```python
from build123d import *

# Parameters (mm, degrees)
BOSS_EXTRUDE1_DEPTH = 5
SKETCH2_R           = 1.5
BOSS_EXTRUDE2_DEPTH = 6
CUT_EXTRUDE1_REACH  = 44.641
SKETCH3_R           = 1.5


with BuildPart() as part:
    # Sketch1 → Boss-Extrude1 (new body)
    with BuildSketch(Plane(origin=(0, 0, 0), x_dir=(1, 0, 0), z_dir=(0, 1, 0))):
        with BuildLine():
            Line((0, 0), (40, 0))
            Line((40, 0), (40, 12.3))
            Line((40, 12.3), (37.05, 12.3))
            ThreePointArc((37.05, 12.3), (36.84816772, 12.496593354), (36.725, 12.75))
            ThreePointArc((36.725, 12.75), (36.593980723, 13.132592289), (36.425, 13.5))
            Line((36.425, 13.5), (35.875, 13.5))
            ThreePointArc((35.875, 13.5), (35.706019277, 13.132592289), (35.575, 12.75))
            ThreePointArc((35.575, 12.75), (35.45183228, 12.496593354), (35.25, 12.3))
            Line((35.25, 12.3), (34.7, 12.3))
            ThreePointArc((34.7, 12.3), (34.49816772, 12.496593354), (34.375, 12.75))
            ThreePointArc((34.375, 12.75), (34.243980723, 13.132592289), (34.075, 13.5))
            Line((34.075, 13.5), (33.525, 13.5))
            ThreePointArc((33.525, 13.5), (33.356019277, 13.132592289), (33.225, 12.75))
            ThreePointArc((33.225, 12.75), (33.10183228, 12.496593354), (32.9, 12.3))
            Line((32.9, 12.3), (32.35, 12.3))
            ThreePointArc((32.35, 12.3), (32.14816772, 12.496593354), (32.025, 12.75))
            ThreePointArc((32.025, 12.75), (31.893980723, 13.132592289), (31.725, 13.5))
            Line((31.725, 13.5), (31.175, 13.5))
            ThreePointArc((31.175, 13.5), (31.006019277, 13.132592289), (30.875, 12.75))
            ThreePointArc((30.875, 12.75), (30.75183228, 12.496593354), (30.55, 12.3))
            Line((30.55, 12.3), (30, 12.3))
            ThreePointArc((30, 12.3), (29.79816772, 12.496593354), (29.675, 12.75))
            ThreePointArc((29.675, 12.75), (29.543980723, 13.132592289), (29.375, 13.5))
            Line((29.375, 13.5), (28.825, 13.5))
            ThreePointArc((28.825, 13.5), (28.656019277, 13.132592289), (28.525, 12.75))
            ThreePointArc((28.525, 12.75), (28.40183228, 12.496593354), (28.2, 12.3))
            Line((28.2, 12.3), (27.65, 12.3))
            ThreePointArc((27.65, 12.3), (27.44816772, 12.496593354), (27.325, 12.75))
            ThreePointArc((27.325, 12.75), (27.193980723, 13.132592289), (27.025, 13.5))
            Line((27.025, 13.5), (26.475, 13.5))
            ThreePointArc((26.475, 13.5), (26.306019277, 13.132592289), (26.175, 12.75))
            ThreePointArc((26.175, 12.75), (26.05183228, 12.496593354), (25.85, 12.3))
            Line((25.85, 12.3), (25.3, 12.3))
            ThreePointArc((25.3, 12.3), (25.09816772, 12.496593354), (24.975, 12.75))
            ThreePointArc((24.975, 12.75), (24.843980723, 13.132592289), (24.675, 13.5))
            Line((24.675, 13.5), (24.125, 13.5))
            ThreePointArc((24.125, 13.5), (23.956019277, 13.132592289), (23.825, 12.75))
            ThreePointArc((23.825, 12.75), (23.70183228, 12.496593354), (23.5, 12.3))
            Line((23.5, 12.3), (22.95, 12.3))
            ThreePointArc((22.95, 12.3), (22.74816772, 12.496593354), (22.625, 12.75))
            ThreePointArc((22.625, 12.75), (22.493980723, 13.132592289), (22.325, 13.5))
            Line((22.325, 13.5), (21.775, 13.5))
            ThreePointArc((21.775, 13.5), (21.606019277, 13.132592289), (21.475, 12.75))
            ThreePointArc((21.475, 12.75), (21.35183228, 12.496593354), (21.15, 12.3))
            Line((21.15, 12.3), (20.6, 12.3))
            ThreePointArc((20.6, 12.3), (20.39816772, 12.496593354), (20.275, 12.75))
            ThreePointArc((20.275, 12.75), (20.143980723, 13.132592289), (19.975, 13.5))
            Line((19.975, 13.5), (19.425, 13.5))
            ThreePointArc((19.425, 13.5), (19.256019277, 13.132592289), (19.125, 12.75))
            ThreePointArc((19.125, 12.75), (19.00183228, 12.496593354), (18.8, 12.3))
            Line((18.8, 12.3), (18.25, 12.3))
            ThreePointArc((18.25, 12.3), (18.04816772, 12.496593354), (17.925, 12.75))
            ThreePointArc((17.925, 12.75), (17.793980723, 13.132592289), (17.625, 13.5))
            Line((17.625, 13.5), (17.075, 13.5))
            ThreePointArc((17.075, 13.5), (16.906019277, 13.132592289), (16.775, 12.75))
            ThreePointArc((16.775, 12.75), (16.65183228, 12.496593354), (16.45, 12.3))
            Line((16.45, 12.3), (15.9, 12.3))
            ThreePointArc((15.9, 12.3), (15.69816772, 12.496593354), (15.575, 12.75))
            ThreePointArc((15.575, 12.75), (15.443980723, 13.132592289), (15.275, 13.5))
            Line((15.275, 13.5), (14.725, 13.5))
            ThreePointArc((14.725, 13.5), (14.556019277, 13.132592289), (14.425, 12.75))
            ThreePointArc((14.425, 12.75), (14.30183228, 12.496593354), (14.1, 12.3))
            Line((14.1, 12.3), (13.55, 12.3))
            ThreePointArc((13.55, 12.3), (13.34816772, 12.496593354), (13.225, 12.75))
            ThreePointArc((13.225, 12.75), (13.093980723, 13.132592289), (12.925, 13.5))
            Line((12.925, 13.5), (12.375, 13.5))
            ThreePointArc((12.375, 13.5), (12.206019277, 13.132592289), (12.075, 12.75))
            ThreePointArc((12.075, 12.75), (11.95183228, 12.496593354), (11.75, 12.3))
            Line((11.75, 12.3), (11.2, 12.3))
            ThreePointArc((11.2, 12.3), (10.99816772, 12.496593354), (10.875, 12.75))
            ThreePointArc((10.875, 12.75), (10.743980723, 13.132592289), (10.575, 13.5))
            Line((10.575, 13.5), (10.025, 13.5))
            ThreePointArc((10.025, 13.5), (9.856019277, 13.132592289), (9.725, 12.75))
            ThreePointArc((9.725, 12.75), (9.60183228, 12.496593354), (9.4, 12.3))
            Line((9.4, 12.3), (8.85, 12.3))
            ThreePointArc((8.85, 12.3), (8.64816772, 12.496593354), (8.525, 12.75))
            ThreePointArc((8.525, 12.75), (8.393980723, 13.132592289), (8.225, 13.5))
            Line((8.225, 13.5), (7.675, 13.5))
            ThreePointArc((7.675, 13.5), (7.506019277, 13.132592289), (7.375, 12.75))
            ThreePointArc((7.375, 12.75), (7.25183228, 12.496593354), (7.05, 12.3))
            Line((7.05, 12.3), (6.5, 12.3))
            ThreePointArc((6.5, 12.3), (6.29816772, 12.496593354), (6.175, 12.75))
            ThreePointArc((6.175, 12.75), (6.043980723, 13.132592289), (5.875, 13.5))
            Line((5.875, 13.5), (5.325, 13.5))
            ThreePointArc((5.325, 13.5), (5.156019277, 13.132592289), (5.025, 12.75))
            ThreePointArc((5.025, 12.75), (4.90183228, 12.496593354), (4.7, 12.3))
            Line((4.7, 12.3), (4.15, 12.3))
            ThreePointArc((4.15, 12.3), (3.94816772, 12.496593354), (3.825, 12.75))
            ThreePointArc((3.825, 12.75), (3.693980723, 13.132592289), (3.525, 13.5))
            Line((3.525, 13.5), (2.975, 13.5))
            ThreePointArc((2.975, 13.5), (2.806019277, 13.132592289), (2.675, 12.75))
            ThreePointArc((2.675, 12.75), (2.55183228, 12.496593354), (2.35, 12.3))
            Line((2.35, 12.3), (1.8, 12.3))
            ThreePointArc((1.8, 12.3), (1.59816772, 12.496593354), (1.475, 12.75))
            ThreePointArc((1.475, 12.75), (1.343980723, 13.132592289), (1.175, 13.5))
            Line((1.175, 13.5), (0.625, 13.5))
            ThreePointArc((0.625, 13.5), (0.456019277, 13.132592289), (0.325, 12.75))
            ThreePointArc((0.325, 12.75), (0.20183228, 12.496593354), (0, 12.3))
            Line((0, 12.3), (0, 0))
        make_face()
    extrude(amount=BOSS_EXTRUDE1_DEPTH)

    # Sketch2 → Boss-Extrude2 (add)
    # profile 1 of 2: a face of its own
    with BuildSketch(Plane.XZ):
        with BuildLine():
            Line((7, -7.5), (3, -7.5))
            ThreePointArc((3, -7.5), (0.5, -5), (3, -2.5))
            Line((3, -2.5), (7, -2.5))
            ThreePointArc((7, -2.5), (9.5, -5), (7, -7.5))
        make_face()
        with Locations(Location((5, -5, 0), (0, 0, 270))):
            Circle(SKETCH2_R, mode=Mode.SUBTRACT)
    # profile 2 of 2: a face of its own
    with BuildSketch(Plane.XZ):
        with BuildLine():
            Line((37, -7.5), (33, -7.5))
            ThreePointArc((33, -7.5), (30.5, -5), (33, -2.5))
            Line((33, -2.5), (37, -2.5))
            ThreePointArc((37, -2.5), (39.5, -5), (37, -7.5))
        make_face()
        with Locations(Location((35, -5, 0), (0, 0, 270))):
            Circle(SKETCH2_R, mode=Mode.SUBTRACT)
    extrude(amount=BOSS_EXTRUDE2_DEPTH)

    # Sketch3 → Cut-Extrude1 (cut, up to next)
    with BuildSketch(Plane.XZ, mode=Mode.PRIVATE) as cut_extrude1_sk1:
        with Locations(Location((35, -5, 0), (0, 0, 270))):
            Circle(SKETCH3_R)
    cut_extrude1_tool1 = extrude(cut_extrude1_sk1.sketch, amount=-CUT_EXTRUDE1_REACH, mode=Mode.PRIVATE) & part.part
    # Sketch3 → Cut-Extrude1 (cut, up to next)
    with BuildSketch(Plane.XZ, mode=Mode.PRIVATE) as cut_extrude1_sk2:
        with Locations(Location((5, -5, 0), (0, 0, 270))):
            Circle(SKETCH3_R)
    cut_extrude1_tool2 = extrude(cut_extrude1_sk2.sketch, amount=-CUT_EXTRUDE1_REACH, mode=Mode.PRIVATE) & part.part
    add(cut_extrude1_tool1.solids().sort_by_distance((35, 0, -5))[0], mode=Mode.SUBTRACT)
    add(cut_extrude1_tool2.solids().sort_by_distance((5, 0, -5))[0], mode=Mode.SUBTRACT)


solid = part.part
```
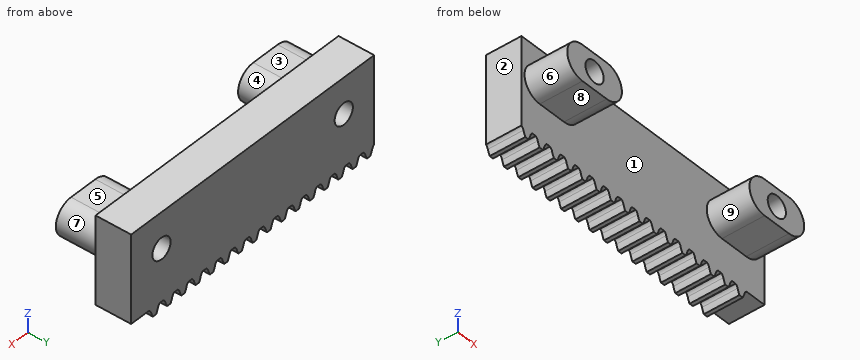
Check sheet for the modelled part. Datum: model origin and axes. Units: mm. Face numbers are marked on the shaded views. A direction names the side the tool comes from. Round coordinates to 2 decimals unless told otherwise and drop trailing zeros. Order: outer loops, then holes, each group sorted by start corner. A loop starts at its lowest first (then second) coordinate and runs counter-clockwise, first axis right, second up. Notation, with made-up numbers: (-27.5, 49) - (-6.5, 49) arc R25 cw to (-6.5, 82) - close; hole circle Ø8 at (39.5, 86). An arc over 180 degrees is marked (long way). Answer as CSV lines item,"result". Start each with the question number.
1) Scan lines: probe 1 along X at (y, z) = (2.55, -5); probe 2 along X at (y, z) = (-3.25, -5); probe 3 along X at (y, z) = (3.25, -6). Record each from-to range of solid material in increasing order.
2) Draft check along X on the marked faces 1, 2, 3 and 4. Enter one of: +X half, -X half, draft (parallel to the pull), parting line (faces both ways), or undercut.
3) Depth check by flat-ended pin: pin 1 (1.5 mm diameter, centred on x = 38, y = 2, fed in from -Z); pin 2 (2 mm diameter, centred on x = 35.5, y = -2.5, fed in from -Z); pin 3 (1.2 mm diameter, centred on x = 4.5, y = -2, fed in from +Z). Enter the tip coordinate at first touch or a pass-through.
4) Section check C-C (z = -10.25). Record the cut outline in (x, y), then the cut area to 3 significant figures.
5) Tool access check on the marked faces 5, 6, 7, 8 and 9. Record the directions out of +Z, -Z, +X, -X, +Y, -Y that give a thin tool (end or side, any length) a straight path to the whole face; none if there is none.
6) Section check A-A (y = -1.5). Record the cut outline in (x, z), then the cut area to 3 significant figures.
7) Section check D-D (x = 37.5). Record the cut outline in (y, z).
8) Section check B-B (z = -5). Record the cut outline in (x, y), then the cut area to 3 significant figures.
Determined:
1,probe 1,"0 to 3.5, 6.5 to 33.5, 36.5 to 40"
1,probe 2,"0.5 to 3.5, 6.5 to 9.5, 30.5 to 33.5, 36.5 to 39.5"
1,probe 3,"0 to 3.88, 6.12 to 33.88, 36.12 to 40"
2,face 1,"undercut"
2,face 2,"-X half"
2,face 3,"draft"
2,face 4,"undercut"
3,pin 1,"z = -12.3"
3,pin 2,"z = -7.5"
3,pin 3,"z = -2.5"
4,outline,"(0, 0) - (40, 0) - (40, 5) - (0, 5) - close"
4,area,"200 mm^2"
5,face 5,"+Z, +X, -X, -Y"
5,face 6,"-X, -Y"
5,face 7,"+X, -Y"
5,face 8,"-Z, +X, -X, -Y"
5,face 9,"-Y"
6,outline,"(3, -7.5) - (7, -7.5) arc R2.5 ccw to (7, -2.5) - (3, -2.5) arc R2.5 ccw to start; (33, -7.5) - (37, -7.5) arc R2.5 ccw to (37, -2.5) - (33, -2.5) arc R2.5 ccw to start; hole circle Ø3 at (5, -5); hole circle Ø3 at (35, -5)"
6,area,"65.1 mm^2"
7,outline,"(-6, -7.45) - (0, -7.45) - (0, -12.3) - (5, -12.3) - (5, 0) - (0, 0) - (0, -2.55) - (-6, -2.55) - close"
8,outline,"(0, 0) - (0.5, 0) - (0.5, -6) - (3.5, -6) - (3.5, 5) - (0, 5) - close; (6.5, -6) - (9.5, -6) - (9.5, 0) - (30.5, 0) - (30.5, -6) - (33.5, -6) - (33.5, 5) - (6.5, 5) - close; (36.5, -6) - (39.5, -6) - (39.5, 0) - (40, 0) - (40, 5) - (36.5, 5) - close"
8,area,"242 mm^2"
